Check sheet for the modelled part. Datum: model origin and axes. Units: mm. A direction names the side the tool comes from. Round coordinates to 2 decimals unless told otherwise and drop trailing zeros. Order: outer loops, then holes, each group sorted by start corner. A loop starts at its lowest first (then second) coordinate and runs counter-clockwise, first axis right, second up. Notation, with made-up numbers: M 23,41.25 L 53,41.25 A27 cw 53,78.25 Z; hole C 85.25,83.25 d9. An arc over 180 degrees is marked long. One line per item, written item: value. Start each with the question number.
(1) Cross-section at B-B, the plane x = 0. Enter the section's corners in (y, z).
(2) Depth check by flat-ended pin: pin 1 Ø2 at (x, z) = (-2.5, -0.5) entering from +Y; pin 2 Ø2 at (x, z) = (-1.5, -4.5) entering from -Y; pin 3 Ø3 at (y, z) = (4.5, -3) entering from +X. Enter the tip coordinate at first touch or a pass-through.
(3) Access from +Z, -Z, +X, -X, +Y, -Y to the whole of each face (thin tool, end or side, straight path). Record for faces 1 (the face through (-3, 0, 0)), 2 (the face through (-0.06, -5.15, -2.12)), 3 (the face through (0.06, 5.15, -2.12)), 4 (the face through (-2.7, 0, -2)).
(4) Cross-section at A-A, the plane y = -1. Enter the section's corners in (x, z).
(5) Thickness scan on L1, parallel to X at y = 2.5, z = -2.25; L2, parallel to Z at x = 2.5, y = 5; L3, parallel to Y at x = 1.5, z = -1.75 (3 decimals). Record the ranges inside material, lowest first.
(6) Cross-section at C-C, the plane z = -2. Enter the section's corners in (x, y), and give its area (3 significant figures).
(7) Cross-section at D-D, the plane z = -4.75. Enter the section's corners in (x, y), and give its area (3 significant figures).
Autodesk Inventor part; units mm, degrees
ref_plane "YZ Plane" through (0, 0, 0) normal (1, 0, 0) x (0, 1, 0)
ref_plane "XZ Plane" through (0, 0, 0) normal (0, 1, 0) x (-1, 0, 0)
ref_plane "XY Plane" through (0, 0, 0) normal (0, 0, 1) x (1, 0, 0)
sketch "Sketch1" plane through (0, 0, 0) normal (0, 0, 1) x (1, 0, 0)
  line L0 (0, -2.45) -> (0, 2.45) construction
  line L1 (4, -2.45) -> (4, 2.45)
  line L2 (-4, 2.45) -> (-4, -2.45)
  arc A0 (-4, -2.45) -> (4, -2.45) centre (0, -2.45) ccw
  arc A1 (4, 2.45) -> (-4, 2.45) centre (0, 2.45) ccw
  point P0 (0, 0)
  dimension "d0" = 2.45
  dimension "d1" = 8
extrude "Extrusion1" add sketch "Sketch1" along normal blind 1.5
sketch "Sketch2" plane through (0, 0, 0) normal (0, 0, -1) x (-1, 0, 0)
  line L0 (-4, -2.45) -> (-4, 2.45)
  arc A0 (-4, -2.45) -> (4, -2.45) centre (0, -2.45) ccw
  line L1 (4, 2.45) -> (4, -2.45)
  arc A1 (4, 2.45) -> (-4, 2.45) centre (0, 2.45) ccw
  line L2 (-2.7, 2.45) -> (-2.7, -2.45)
  arc A2 (-2.7, -2.45) -> (2.7, -2.45) centre (0, -2.45) ccw
  line L3 (2.7, -2.45) -> (2.7, 2.45)
  arc A3 (2.7, 2.45) -> (-2.7, 2.45) centre (0, 2.45) ccw
  point P0 (0, 0)
  dimension "d4" = 1.3
extrude "Extrusion2" add sketch "Sketch2" along normal blind 5.3 contours A3 L3 A2 L2
fillet "Fillet1" radius 1 4 edges at (2.7, 0, -5.3) (0, -5.15, -5.3) (-2.7, 0, -5.3) (0, 5.15, -5.3)
properties part number "LCDButton" material "ABS Plastic"
Values found:
1. outline: M -6.45,0 L -5.15,0 L -5.15,-4.3 A1 ccw -4.15,-5.3 L 4.15,-5.3 A1 ccw 5.15,-4.3 L 5.15,0 L 6.45,0 L 6.45,1.5 L -6.45,1.5 Z
2. pin 1: y = 6.1
2. pin 2: y = -5.1
2. pin 3: x = 2.64
3. face 1: -Z
3. face 2: -Z, -Y
3. face 3: -Z, +Y
3. face 4: -Z, -X, +Y, -Y
4. outline: M -4,0 L -2.7,0 L -2.7,-4.3 A1 ccw -1.7,-5.3 L 1.7,-5.3 A1 ccw 2.7,-4.3 L 2.7,0 L 4,0 L 4,1.5 L -4,1.5 Z
5. L1: -2.7 to 2.7
5. L2: 0 to 1.5
5. L3: -4.695 to 4.695
6. outline: M -2.7,-2.45 A2.7 ccw 2.7,-2.45 L 2.7,2.45 A2.7 ccw -2.7,2.45 Z
6. area: 49.4 mm^2
7. outline: M -2.59,-2.45 A2.59 ccw 2.59,-2.45 L 2.59,2.45 A2.59 ccw -2.59,2.45 Z
7. area: 46.5 mm^2
